The listing builds one solid part. Answer for the finished solid, in the listing's coordinates (mm). Face numbers are marked on the shaded views. A direction names the side the tool comes from. Round coordinates to 2 decimals unless told otherwise and drop trailing zeros. Loops run counter-clockwise (first coordinate to the right, second up) from the corner with the lowest first, then second, coordinate; pieces in that order, holes last. Notation, with made-up numbers: (-33.5, 54.25) - (-13.5, 54.25) arc R16 cw to (-13.5, 65.25) - close; hole circle Ø3 at (53.5, 53). An arc over 180 degrees is marked (long way). One line per item, written item: value.
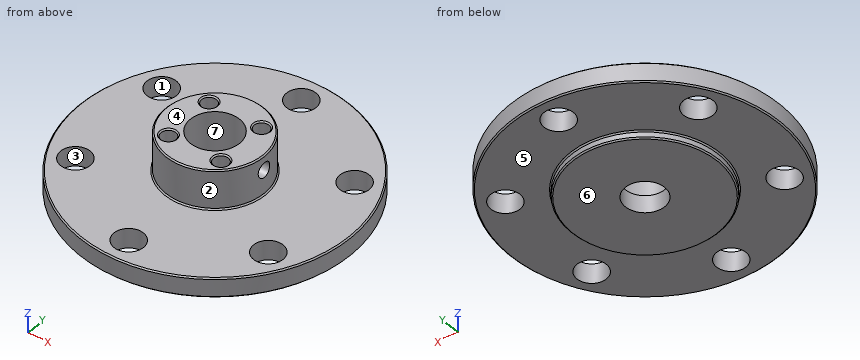
```python
from build123d import *

# Parameters (mm, degrees)
SKETCH1_R           = 27.5
SKETCH1_R_2         = 3
BOSS_EXTRUDE1_DEPTH = 4
SKETCH2_R           = 10
BOSS_EXTRUDE2_DEPTH = 8
SKETCH3_R           = 15
BOSS_EXTRUDE3_DEPTH = 1.5
SKETCH4_R           = 1.5
CUT_EXTRUDE2_DEPTH  = 6
CUT_EXTRUDE3_START  = 10
SKETCH5_R           = 1.5
CUT_EXTRUDE3_DEPTH  = 3.5
SKETCH6_R           = 5
CUT_EXTRUDE4_DEPTH  = 10
SKETCH7_R           = 4
CUT_EXTRUDE5_DEPTH  = 42.167341458
CHAMFER1_SIZE       = 0.25
CHAMFER2_SIZE       = 0.25


with BuildPart() as part:
    # Sketch1 → Boss-Extrude1 (new body)
    with BuildSketch(Plane.XY):
        Circle(SKETCH1_R)
        with Locations((0, 22.5)):
            Circle(SKETCH1_R_2, mode=Mode.SUBTRACT)
        with Locations((19.485571585, 11.25)):
            Circle(SKETCH1_R_2, mode=Mode.SUBTRACT)
        with Locations((19.485571585, -11.25)):
            Circle(SKETCH1_R_2, mode=Mode.SUBTRACT)
        with Locations((0, -22.5)):
            Circle(SKETCH1_R_2, mode=Mode.SUBTRACT)
        with Locations((-19.485571585, -11.25)):
            Circle(SKETCH1_R_2, mode=Mode.SUBTRACT)
        with Locations((-19.485571585, 11.25)):
            Circle(SKETCH1_R_2, mode=Mode.SUBTRACT)
    extrude(amount=BOSS_EXTRUDE1_DEPTH)

    # Sketch2 → Boss-Extrude2 (add)
    with BuildSketch(Plane.XY.offset(4)):
        Circle(SKETCH2_R)
    extrude(amount=BOSS_EXTRUDE2_DEPTH)

    # Sketch3 → Boss-Extrude3 (add)
    with BuildSketch(Plane(origin=(0, 0, 0), x_dir=(-1, 0, 0), z_dir=(0, 0, -1))):
        with Locations(Location((0, 0, 0), (0, 0, 180))):
            Circle(SKETCH3_R)
    extrude(amount=BOSS_EXTRUDE3_DEPTH)

    # Sketch4 → Cut-Extrude2 (cut)
    with BuildSketch(Plane.XY.offset(12)):
        with Locations((-5.303300859, 5.303300859)):
            Circle(SKETCH4_R)
        with Locations((5.303300859, 5.303300859)):
            Circle(SKETCH4_R)
        with Locations((5.303300859, -5.303300859)):
            Circle(SKETCH4_R)
        with Locations((-5.303300859, -5.303300859)):
            Circle(SKETCH4_R)
    extrude(amount=-CUT_EXTRUDE2_DEPTH, mode=Mode.SUBTRACT)

    # Sketch5 → Cut-Extrude3 (cut)
    with BuildSketch(Plane(origin=(0, 0, 0), x_dir=(0, 0, -1), z_dir=(1, 0, 0)).offset(CUT_EXTRUDE3_START)):
        with Locations((-9, 0)):
            Circle(SKETCH5_R)
    cut_extrude3 = extrude(amount=-CUT_EXTRUDE3_DEPTH, mode=Mode.SUBTRACT)

    # Mirror1: Cut-Extrude3 across plane
    add(cut_extrude3.mirror(Plane(origin=(0, 0, 0), x_dir=(0, 0, 1), z_dir=(1, 0, 0))), mode=Mode.SUBTRACT)

    # Sketch6 → Cut-Extrude4 (cut)
    with BuildSketch(Plane.XY.offset(12)):
        Circle(SKETCH6_R)
    extrude(amount=-CUT_EXTRUDE4_DEPTH, mode=Mode.SUBTRACT)

    # Sketch7 → Cut-Extrude5 (cut, through all)
    with BuildSketch(Plane(origin=(0, 0, -1.5), x_dir=(-1, 0, 0), z_dir=(0, 0, -1))):
        Circle(SKETCH7_R)
    extrude(amount=-CUT_EXTRUDE5_DEPTH, mode=Mode.SUBTRACT)

    # Chamfer1
    chamfer1_edges = [part.edges().sort_by_distance(p)[0] for p in [
        (-6.803300859, -5.303300859, 12),
        (3.803300859, -5.303300859, 12),
        (3.803300859, 5.303300859, 12),
        (-6.803300859, 5.303300859, 12),
    ]]
    chamfer(chamfer1_edges, length=CHAMFER1_SIZE)

    # Chamfer2
    chamfer2_edges = [part.edges().sort_by_distance(p)[0] for p in [
        (-27.5, 0, 0),
        (-10, 0, 4),
        (-10, 0, 12),
        (-15, 0, 0),
        (-15, 0, -1.5),
        (-27.5, 0, 4),
    ]]
    chamfer(chamfer2_edges, length=CHAMFER2_SIZE)


solid = part.part
```
1) Each of these flat-tipped pins is pushed along its axis until it touches: pin 1 Ø3.5 at (y, z) = (0, 9) entering from +X; pin 2 Ø6 at (x, y) = (-10.5, -20) entering from -Z; pin 3 Ø2.5 at (y, z) = (0, 9) entering from +X. Where does it stop, or does it pass through?
Final values:
pin 1: x = 10
pin 2: z = 0
pin 3: x = 6.5
2) Consider L1, parallel to Y at x = 0, z = 2.75; L2, parallel to Y at x = 0, z = 4.75; L3, parallel to Z at x = 21.5, y = -8. Determine where each line is inside the solid, lowest interval first.
Final values:
L1: -27.5 to -25.5, -19.5 to -5, 5 to 19.5, 25.5 to 27.5
L2: -10 to -5, 5 to 10
L3: 0 to 4
3) A cutting plane is placed at A-A on z = 9. Give the vertices of the cut face in (x, y).
Final values:
outline: (-9.89, -1.5) arc R10 ccw to (9.89, -1.5) - (6.5, -1.5) - (6.5, 1.5) - (9.89, 1.5) arc R10 ccw to (-9.89, 1.5) - (-6.5, 1.5) - (-6.5, -1.5) - close; hole circle Ø3 at (-5.3, -5.3); hole circle Ø3 at (-5.3, 5.3); hole circle Ø10 at (0, 0); hole circle Ø3 at (5.3, -5.3); hole circle Ø3 at (5.3, 5.3)
4) A cutting plane is placed at C-C on z = 5.25. Give the vertices of the cut face in (x, y), and give its area (3 significant figures).
Final values:
outline: circle Ø20 at (0, 0); hole circle Ø10 at (0, 0)
area: 236 mm2
5) For a pull along X with two mould halves and no side action, classify the marked faces 1, 2, 3 and 4 as released by +X, released by -X, zero draft, split by the parting line, or undercut.
Final values:
face 1: undercut
face 2: split by the parting line
face 3: undercut
face 4: zero draft
6) A cutting plane is placed at B-B on x = -17.5. Give the number of separate pieces and of enclosed holes in the cut face, and give its area (3 significant figures).
Final values:
separate pieces: 3
enclosed holes: 0
area: 134 mm2
7) For the marked faces 5, 6 and 7, determine the directions among +Z, -Z, +X, -X, +Y, -Y from which every point of the face is accessible in a straight line to the end or side of a thin tool.
Final values:
face 5: -Z
face 6: -Z, +X, -X, +Y, -Y
face 7: +Z
